from build123d import *

# Parameters (mm, degrees)
CUT_EXTRUDE_1_DEPTH      = 96.582051988
CUT_EXTRUDE_1_DEPTH_BACK = 96.582051988
FILLET_1_R               = 0.25
SKETCH_4_R               = 1.25
CUT_EXTRUDE_2_DEPTH      = 85.125637832
SKETCH_5_R               = 2.5
EXTRUDE_1_DEPTH          = 6
SKETCH_6_W               = 7
SKETCH_6_H               = 13.635845178
CUT_EXTRUDE_3_DEPTH      = 104.240069036


with BuildPart() as part:
    # 草图1 → 旋转1 (revolve)
    with BuildSketch(Plane(origin=(0, -42.25, 0), x_dir=(1, 0, 0), z_dir=(0, 1, 0)), mode=Mode.PRIVATE) as revolve_1_sk:
        Polygon((57.25, -47), (57.25, -53), (57.25, -58.375), (60.489565186, -58.375), (60.489565186, -47), align=None)
    revolve(revolve_1_sk.sketch.rotate(Axis((57.25, -42.25, 47), (0, 0, 1)), 180), axis=Axis((57.25, -42.25, 47), (0, 0, 1)))

    # 草图2 → 切除-拉伸1 (cut, two sides: drawn at the far end of the back side and taken through both)
    with BuildSketch(Plane(origin=(0, 0, 0), x_dir=(0, 0, -1), z_dir=(1, 0, 0)).offset(-CUT_EXTRUDE_1_DEPTH_BACK)):
        Polygon((-48.25, -42.25), (-53, -42.25), (-54.875, -45.5), (-45.95593144, -45.5), (-45.95593144, -39), (-47, -39), align=None)
    extrude(amount=CUT_EXTRUDE_1_DEPTH + CUT_EXTRUDE_1_DEPTH_BACK, mode=Mode.SUBTRACT)

    # 圆角1
    fillet_1_edges = [part.edges().sort_by_distance(p)[0] for p in [
        (57.250000001, -39.010434814, 47.00401339),
        (54.010434814, -42.25, 50.625),
        (57.249999966, -45.489565186, 54.868979915),
        (60.489565186, -42.25, 50.625),
    ]]
    fillet(fillet_1_edges, radius=FILLET_1_R)

    # 草图4 → 切除-拉伸2 (cut, through all)
    with BuildSketch(Plane.XZ.offset(42.25)):
        with Locations(Location((57.25, 50.75, 0), (0, 0, 270))):
            Circle(SKETCH_4_R)
    extrude(amount=-CUT_EXTRUDE_2_DEPTH, mode=Mode.SUBTRACT)

    # 草图5 → 凸台-拉伸1 (add, symmetric)
    with BuildSketch(Plane(origin=(57.25, 0, 0), x_dir=(0, 0, -1), z_dir=(1, 0, 0))):
        with BuildLine():
            Line((-64.5, -45.489565186), (-58.375, -45.489565186))
            Line((-58.375, -45.489565186), (-58.375, -39.010434814))
            Line((-58.375, -39.010434814), (-64.5, -39.010434814))
            ThreePointArc((-64.5, -39.010434814), (-67.739565186, -42.25), (-64.5, -45.489565186))
        make_face()
        with Locations((-64.5, -42.25)):
            Circle(SKETCH_5_R, mode=Mode.SUBTRACT)
    extrude(amount=EXTRUDE_1_DEPTH, both=True)

    # 草图6 → 切除-拉伸3 (cut, through all)
    with BuildSketch(Plane(origin=(0, 0, 0), x_dir=(1, 0, 0), z_dir=(0, 1, 0))):
        with Locations((57.25, -67.692922589)):
            Rectangle(SKETCH_6_W, SKETCH_6_H)
    extrude(amount=-CUT_EXTRUDE_3_DEPTH, mode=Mode.SUBTRACT)


solid = part.part
Model file for the job. Use its own axes, mm. A direction names the side the tool comes from. Round coordinates to 2 decimals unless told otherwise and drop trailing zeros. Order: outer loops, then holes, each group sorted by start corner. A loop starts at its lowest first (then second) coordinate and runs counter-clockwise, first axis right, second up. Notation, with made-up numbers: M 47.5,-1.75 L 59.5,-1.75 A12 cw 59.5,16.25 Z; hole C 36.5,-27.75 d10. An arc over 180 degrees is marked long. Write each question's results on one line, items separated by ' | '. Start each with the question number.
(1) Saw through at C-C, the plane z = 50.75. Give the cut face in (x, y).
(2) Saw through at A-A, the plane z = 62.5. Give the cut face in (x, y), then the cut area to 3 significant figures.
(3) Two-plate mould, pull along Y, no slides. Class faces 4 (the face through (61.98, -43.21, 62.19)), 5 (the face through (57, -45.49, 60)), 6 (the face through (57.63, -40.65, 49.56)): pulls with the +Y half, pulls with the -Y half, needs draft (parallel to the pull), parting line crosses it, or undercut.
(4) Drop flat-ended pins along their axis: pin 1 (1 mm diameter, centred on x = 54.5, y = -40.5, fed in from -Z); pin 2 (1.4 mm diameter, centred on x = 56, z = 52, fed in from -Y). Give the stop position or say it passes through.
(5) Saw through at D-D, the plane y = -41.75. State how many separate pieces and enclosed holes the cut face has, then the cut area to 3 significant figures.
(6) Probe probe 1 along Z at (x, y) = (62.3, -42.25) (3 decimals); probe 2 along X at (y, z) = (-39.5, 65.5); probe 3 along Y at (x, z) = (52.9, 64.5). List the from-to ranges inside material, lowest first. Write a range as from..to.
(7) Saw through at B-B, the plane x = 53. Give the cut face in (y, z) (3 decimals), then the cut area to 3 significant figures.
(8) Which spindle directions (+Z, -Z, +X, -X, +Y, -Y) get a long thin tool onto all of the face, cutting with end or side? Do faces 1 (the face through (53.75, -41, 62)), 2 (the face through (56.5, -42.25, 49.5)), 3 (the face through (58, -39.1, 54)). Say none if no direction does.
Established:
1) outline: M 54.02,-41.98 A0.25 ccw 54.27,-42.25 L 56,-42.25 L 56,-39.26 A3.24 ccw Z; M 58.5,-42.25 L 60.23,-42.25 A0.25 ccw 60.48,-41.98 A3.24 ccw 58.5,-39.26 Z
2) outline: M 51.25,-45.49 L 53.75,-45.49 L 53.75,-43.75 L 51.25,-43.75 Z; M 51.25,-40.75 L 53.75,-40.75 L 53.75,-39.01 L 51.25,-39.01 Z; M 60.75,-45.49 L 63.25,-45.49 L 63.25,-43.75 L 60.75,-43.75 Z; M 60.75,-40.75 L 63.25,-40.75 L 63.25,-39.01 L 60.75,-39.01 Z | area: 17.4 mm^2
3) face 4: undercut | face 5: pulls with the -Y half | face 6: needs draft
4) pin 1: stops at z = 47.51 | pin 2: stops at y = -42.25
5) separate pieces: 3 | enclosed holes: 1 | area: 101 mm^2
6) probe 1: z = 58.375..62, 67..67.74 | probe 2: x = 51.25..53.75, 60.75..63.25 | probe 3: y = -45.49..-44.75, -39.75..-39.01
7) outline: M -45.49,58.375 L -39.01,58.375 L -39.01,64.5 A3.24 ccw -45.49,64.5 Z; hole C -42.25,64.5 d5 | area: 36.5 mm^2
8) face 1: +Z, +Y, -Y | face 2: -Z, +X, -X, -Y | face 3: -Z
